Build history of the part. All positions in model axes, mm. Give positions to 0.01 mm unless a question says otherwise; leave off trailing zeros. Write each loop counter-clockwise with the first axis right and the second up, starting at its lowest first coordinate (ties: lowest second). Pieces come first, ordered by that corner, then holes. Notation, with made-up numbers: (-22.5, 33) -> (6.5, 33) arc R28 ccw to (6.5, 58) -> close; hole circle Ø7 at (-33, -27.5). An arc over 180 degrees is marked (long way). Put each result on its own line as item: value. Start each with the question number.
Item 1: Drill centre lines: line 1 along Y through (x, z) = (0, 0.95) (3 decimals); line 2 along X through (y, z) = (-54.5, 0.95) (3 decimals); line 3 along X through (y, z) = (-64.5, 2.8) (3 decimals). Where is each one in solid material? Low to high.
Item 2: Slice it at A-A, the plane y = -100. List the corners of the cut face in (x, z) (3 decimals).
Item 3: Slice it at C-C, the plane y = 0. List the corners of the cut face in (x, z) (3 decimals), plus the area to 3 significant figures.
Item 4: Slice it at B-B, the plane z = 0.5. Give the number of separate pieces and of enclosed holes in the cut face, plus the area to 3 significant figures.
Item 5: Flat gauge pins, fed straight in: pin 1 Ø1 at (x, z) = (-21, 1.5) entering from -Y; pin 2 Ø6 at (x, y) = (38.17, -38.17) entering from +Z (3 decimals); pin 3 Ø1 at (y, z) = (-93.5, 1.5) entering from +X (3 decimals); pin 4 Ø1.5 at (y, z) = (-76, 2.5) entering from -X. Where does each tip first touch, or does it go through?
Item 6: Slice it at D-D, the plane y = -82. List the corners of the cut face in (x, z) (3 decimals).
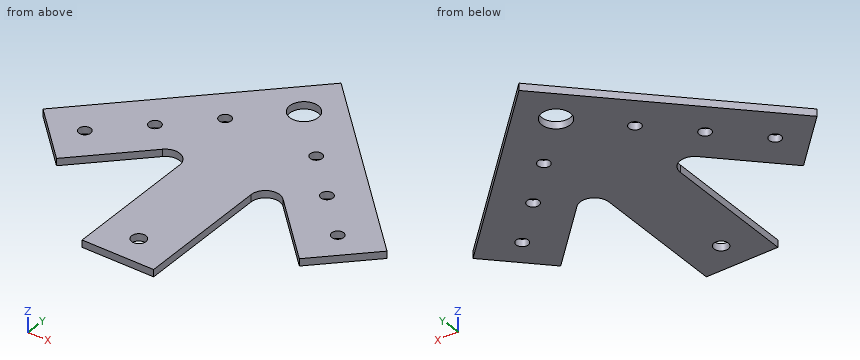
Autodesk Inventor part; units mm, degrees
ref_plane "YZ Plane" through (0, 0, 0) normal (1, 0, 0) x (0, 1, 0)
ref_plane "XZ Plane" through (0, 0, 0) normal (0, 1, 0) x (-1, 0, 0)
ref_plane "XY Plane" through (0, 0, 0) normal (0, 0, 1) x (1, 0, 0)
sketch "Sketch1" plane through (0, 0, 0) normal (0, 0, 1) x (1, 0, 0)
  line L0 (-53.8815, -76.3322) -> (-15.875, -38.3256)
  line L1 (-53.8815, -76.3322) -> (-76.3322, -53.8815)
  line L2 (-76.3322, -53.8815) -> (0, 22.4506)
  line L3 (53.8815, -76.3322) -> (15.875, -38.3256)
  line L4 (53.8815, -76.3322) -> (76.3322, -53.8815)
  line L5 (76.3322, -53.8815) -> (0, 22.4506)
  line L6 (-106.865, 0) -> (106.865, 0)
  line L7 (-15.875, -38.3256) -> (-15.875, -112.7)
  line L8 (-15.875, -112.7) -> (15.875, -112.7)
  line L9 (15.875, -112.7) -> (15.875, -38.3256)
  circle A0 centre (0, -100) radius 3.175
  line L10 (0, -139.7301) -> (0, 49.4808)
  circle A1 centre (0, 0) radius 6.35
  point P0 (0, -112.7)
  dimension "d13" = 31.75
  dimension "d38" = 100
  dimension "d39" = 45
  dimension "d41" = 15.875
  dimension "d43" = 112.7
  dimension "d44" = 12.7
  dimension "d47" = 15.875
  dimension "d48" = 76.2
extrude "Extrusion1" add sketch "Sketch1" along normal blind 3.175 contours L1 L2 L6 A1 L10 A0 L8 L7 L0 | L2 L10 A1 L6 | L10 A0 A1 L6 L5 L4 L3 L9 L8 | L5 L6 A1 L10
sketch "Sketch2" plane through (0, 0, 3.175) normal (0, 0, 1) x (1, 0, 0)
  line L0 (-76.3322, -53.8815) -> (-53.8815, -76.3322)
  line L1 (-65.1069, -65.1069) -> (14.4203, 14.4203)
  line L2 (53.8815, -76.3322) -> (76.3322, -53.8815)
  line L3 (76.3322, -53.8815) -> (0, 22.4506)
  line L4 (0, 22.4506) -> (-76.3322, -53.8815)
  line L5 (-76.3322, -53.8815) -> (-53.8815, -76.3322)
  line L6 (-53.8815, -76.3322) -> (-15.875, -38.3256)
  line L7 (15.875, -38.3256) -> (53.8815, -76.3322)
  circle A0 centre (-56.1266, -56.1266) radius 2.65
  circle A1 centre (-38.1661, -38.1661) radius 2.65
  circle A2 centre (-20.2056, -20.2056) radius 2.65
  line L8 (-15.875, -38.3256) -> (-15.875, -112.7)
  line L9 (-15.875, -112.7) -> (15.875, -112.7)
  line L10 (15.875, -112.7) -> (15.875, -38.3256)
  point P0 (0, 0)
  dimension "d17" = 5.3
  dimension "d18" = 12.7
  dimension "d21" = 25.4
extrude "Extrusion2" cut sketch "Sketch2" against normal blind 3.175 contours A0 L1 | L1 A0 | A2 L1 | L1 A2 | A1 L1 | L1 A1
mirror "Mirror1" about plane through (0, 0, 0) normal (1, 0, 0) of "Extrusion2"
fillet "Fillet3" radius 6.35 2 edges at (-15.875, -38.3256, 1.5875) (15.875, -38.3256, 1.5875)
equation "\"d41\" = 0.5 * d13"
equation "\"d15\" = plateThickness"
equation "\"d17\" = boltDiameter"
equation "\"d26\" = plateThickness"
equation "\"topDiameter\" = 25"
equation "\"shaftLength\" = 76.2"
equation "\"bearingDiameter\" = 28.62"
equation "\"plateThickness\" = 3.175"
equation "\"theta12\" = 100deg"
equation "\"boltDiameter\" = 5.3"
equation "\"gearboxLength\" = 101.6"
equation "\"boltedLength\" = 76.2"
equation "\"innerBoltSpacing\" = 12.7"
equation "\"outerBoltSpacing\" = 12.7"
properties part number "CH-1-HipPivotPlate" material "Aluminum 6061"
Values follow:
1. line 1: -112.7 to -103.175, -96.825 to -6.35, 6.35 to 22.451
1. line 2: -75.714 to -58.219, -54.035 to -32.049, -15.875 to 15.875, 32.049 to 54.035, 58.219 to 75.714
1. line 3: -65.714 to -42.049, -15.875 to 15.875, 42.049 to 65.714
2. outline: (-15.875, 0) -> (-3.175, 0) -> (-3.175, 3.175) -> (-15.875, 3.175) -> close; (3.175, 0) -> (15.875, 0) -> (15.875, 3.175) -> (3.175, 3.175) -> close
3. outline: (-22.451, 0) -> (-6.35, 0) -> (-6.35, 3.175) -> (-22.451, 3.175) -> close; (6.35, 0) -> (22.451, 0) -> (22.451, 3.175) -> (6.35, 3.175) -> close
3. area: 102 mm2
4. separate pieces: 1
4. enclosed holes: 8
4. area: 8,270 mm2
5. pin 1: y = -47.54
5. pin 2: z = 3.175
5. pin 3: x = 15.875
5. pin 4: x = -54.96
6. outline: (-15.875, 0) -> (15.875, 0) -> (15.875, 3.175) -> (-15.875, 3.175) -> close
